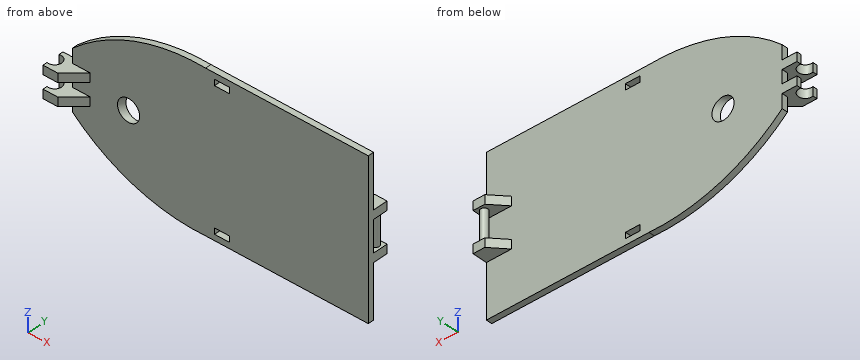
from build123d import *

# Parameters (mm, degrees)
BOSS_EXTRUDE1_DEPTH = 4
BOSS_EXTRUDE2_START = -45
BOSS_EXTRUDE2_DEPTH = 3
BOSS_EXTRUDE3_START = -39
BOSS_EXTRUDE3_DEPTH = 3
BOSS_EXTRUDE4_REACH = 221.731
SKETCH6_R           = 2.5
SKETCH7_W           = 10
SKETCH7_H           = 4
CUT_EXTRUDE1_DEPTH  = 10
SKETCH8_R           = 7.5


with BuildPart() as part:
    # Sketch1 → Boss-Extrude1 (new body)
    with BuildSketch(Plane(origin=(0, 0, 0), x_dir=(1, 0, 0), z_dir=(0, 1, 0))):
        with BuildLine():
            Line((-110, 0), (0, 0))
            Line((0, 0), (0, -105))
            Line((0, -105), (-110, -105))
            ThreePointArc((-110, -105), (-158.232963684, -97.702822508), (-200, -72.5))
            Line((-200, -72.5), (-200, -32.5))
            ThreePointArc((-200, -32.5), (-158.232963684, -7.297177492), (-110, 0))
        make_face()
    extrude(amount=BOSS_EXTRUDE1_DEPTH)

    # Sketch2 → Boss-Extrude2 (add, symmetric)
    with BuildSketch(Plane.XY.offset(105).offset(BOSS_EXTRUDE2_START)):
        with BuildLine():
            Line((-200, 4), (-210, 4))
            Line((-210, 4), (-210, 1))
            ThreePointArc((-210, 1), (-204.2, -3.5), (-210, -8))
            Line((-210, -8), (-210, -11))
            Line((-210, -11), (-200, -11))
            Line((-200, -11), (-188, 0))
            Line((-188, 0), (-200, 4))
        make_face()
    boss_extrude2 = extrude(amount=BOSS_EXTRUDE2_DEPTH, both=True)

    # Mirror1: Boss-Extrude2 across plane
    add(boss_extrude2.mirror(Plane.XY.offset(52.5)))

    # Sketch5 → Boss-Extrude3 (add, symmetric)
    with BuildSketch(Plane.XY.offset(105).offset(BOSS_EXTRUDE3_START)):
        Polygon((-16.979807258, 4), (-7.979807258, 14), (0, 14), (0, 4), align=None)
    boss_extrude3 = extrude(amount=BOSS_EXTRUDE3_DEPTH, both=True)

    # Mirror4: Boss-Extrude3 across plane
    add(boss_extrude3.mirror(Plane.XY.offset(52.5)))

    # Sketch6 → Boss-Extrude4 (add, up to next)
    with BuildSketch(Plane.XY.offset(42), mode=Mode.PRIVATE) as boss_extrude4_sk1:
        with Locations(Location((-4, 10, 0), (0, 0, 180))):
            Circle(SKETCH6_R)
    boss_extrude4_tool1 = extrude(boss_extrude4_sk1.sketch, amount=BOSS_EXTRUDE4_REACH, mode=Mode.PRIVATE) - part.part
    add(boss_extrude4_tool1.solids().sort_by_distance((-4, 10, 42))[0])

    # Sketch7 → Cut-Extrude1 (cut)
    with BuildSketch(Plane(origin=(0, 4, 0), x_dir=(1, 0, 0), z_dir=(0, 1, 0))):
        with Locations((-99, -99)):
            Rectangle(SKETCH7_W, SKETCH7_H)
    cut_extrude1 = extrude(amount=-CUT_EXTRUDE1_DEPTH, mode=Mode.SUBTRACT)

    # Mirror5: Cut-Extrude1 across plane
    add(cut_extrude1.mirror(Plane.XY.offset(52.5)), mode=Mode.SUBTRACT)

    # Cut-Sweep1: sweep along a path in Sketch9
    with BuildLine(Plane.XY.offset(52.5)) as cut_sweep1_path:
        Line((-160, 4), (-163.867437875, -3.466183031))
    # Sketch8 → Cut-Sweep1 (sweep, cut)
    with BuildSketch(Plane(origin=(0, 4, 0), x_dir=(1, 0, 0), z_dir=(0, 1, 0))):
        with Locations((-160, -52.5)):
            Circle(SKETCH8_R)
    sweep(path=cut_sweep1_path.line, mode=Mode.SUBTRACT)


solid = part.part
Design review of the part built by this model. Coordinates are the model's own, in mm. Round coordinates to 2 decimals unless told otherwise and drop trailing zeros. Order: outer loops, then holes, each group sorted by start corner. A loop starts at its lowest first (then second) coordinate and runs counter-clockwise, first axis right, second up. Notation, with made-up numbers: M -3,-9 L 15,-9 A17 cw 15,5 Z; hole C 20.5,-23.75 d3. An arc over 180 degrees is marked long. Answer as CSV lines item,"result". Start each with the question number.
1) Add section D-D (z = 27.5). Give the boundary of the cut face in (x, y).
2) Add section B-B (y = -3.5). Give the boundary of the cut face in (x, z).
3) Wall thickness on line 1 along Z through (x, y) = (-198.5, -3.75); line 2 along Y through (x, z) = (-142.5, 5.5); line 3 along X through (y, z) = (-3.5, 58.4): over which ranges is each line inside the solid? List them lowest first. Write a range as [from, to].
4) For pin 1 Ø5 at (x, y) = (-11.5, 9.5) entering from +Z; pin 2 Ø1.2 at (x, y) = (-98.5, 2) entering from -Z; pin 3 Ø8 at (y, z) = (8.5, 24.5) entering from -X; pin 4 Ø11 at (x, y) = (-11, 7) entering from +Z, all flat-tipped, find the tip position at first contact; note any pin that passes through.
5) Add section C-C (y = 10). Give the boundary of the cut face in (x, z), then the cut area to 3 significant figures.
6) Add section A-A (x = -4). Give the boundary of the cut face in (y, z).
Resolved:
1,outline,"M -194.17,0 L 0,0 L 0,4 L -194.17,4 Z"
2,outline,"M -204.2,42 L -191.82,42 L -191.82,48 L -204.2,48 Z; M -204.2,57 L -191.82,57 L -191.82,63 L -204.2,63 Z"
3,line 1,"[42, 48], [57, 63]"
3,line 2,"[0, 4]"
3,line 3,"[-204.2, -191.82]"
4,pin 1,"z = 69"
4,pin 2,"z = 0"
4,pin 3,"through"
4,pin 4,"z = 105"
5,outline,"M -11.58,36 L 0,36 L 0,42 L -1.5,42 L -1.5,63 L 0,63 L 0,69 L -11.58,69 L -11.58,63 L -6.5,63 L -6.5,42 L -11.58,42 Z"
5,area,"244 mm^2"
6,outline,"M 0,0 L 4,0 L 4,36 L 14,36 L 14,42 L 12.5,42 L 12.5,63 L 14,63 L 14,69 L 4,69 L 4,105 L 0,105 Z; hole M 4,42 L 7.5,42 L 7.5,63 L 4,63 Z"
